Answer from the drawing. Dimensions are ordinates in mm from the lowest x, y and z of the part. Coordinates: 2 decimals unless noted, no trailing zeros. Write each loop counter-clockwise with the first axis right and the second up, starting at its lowest first coordinate (ties: lowest second). Pieces come first, ordered by that corner, then holes. Notation, with made-up numbers: (89, 11.25) -> (105, 11.25) arc R27 ccw to (105, 27.25) -> close; hole circle Ø11 at (-34.5, -31). An arc over 180 degrees is marked (long way). Return JSON: item names as keys, results as strings.
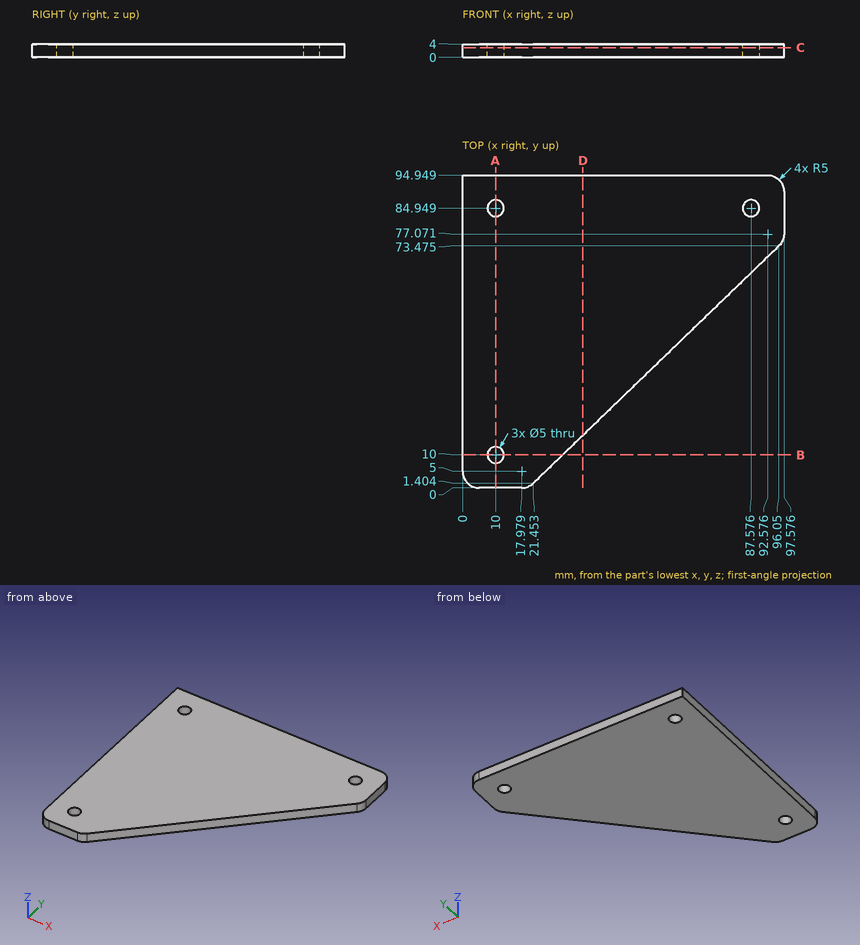
1. Flat-ended cylindrical pins translate along their axes: pin 1 Ø1.5 at (y, z) = (76, 2) entering from -X; pin 2 Ø2 at (y, z) = (51, 1) entering from +X. Find the tip coordinate at first contact, or state that the pin passes through.
Taken from the geometry:
{"pin 1": "stops at x = 0", "pin 2": "stops at x = 73.82"}
2. The part is cut by section C-C (z = 2.9). Count the separate pieces of the cut face and the enclosed holes in it, then the cut area to 3 significant figures.
Taken from the geometry:
{"separate pieces": "1", "enclosed holes": "3", "area": "6,290 mm2"}
3. The part is cut by section B-B (y = 10). Determine the outline of the cut face in (x, z), then the cut area to 3 significant figures.
Taken from the geometry:
{"outline": "(0, 0) -> (7.5, 0) -> (7.5, 4) -> (0, 4) -> close; (12.5, 0) -> (30.35, 0) -> (30.35, 4) -> (12.5, 4) -> close", "area": "101 mm2"}
4. The part is cut by section A-A (x = 10). Determine the outline of the cut face in (y, z).
Taken from the geometry:
{"outline": "(0, 0) -> (7.5, 0) -> (7.5, 4) -> (0, 4) -> close; (12.5, 0) -> (82.45, 0) -> (82.45, 4) -> (12.5, 4) -> close; (87.45, 0) -> (94.95, 0) -> (94.95, 4) -> (87.45, 4) -> close"}
5. Consider L1, parallel to Y at x = 10, z = 2.05; L2, parallel to X at y = 84.5, z = 0.7 (1 decimal); L3, parallel to Y at x = 8, z = 0.5. Determine where each line is inside the solid, lowest interval first.
Taken from the geometry:
{"L1": "y = 0 to 7.5, 12.5 to 82.45, 87.45 to 94.95", "L2": "x = 0 to 7.5, 12.5 to 85.1, 90 to 97.6", "L3": "y = 0 to 8.5, 11.5 to 83.45, 86.45 to 94.95"}
6. The part is cut by section D-D (x = 36.5). Determine the outline of the cut face in (y, z), then the cut area to 3 significant figures.
Taken from the geometry:
{"outline": "(15.94, 0) -> (94.95, 0) -> (94.95, 4) -> (15.94, 4) -> close", "area": "316 mm2"}
